Autodesk Inventor part; units mm, degrees
ref_plane "YZ Plane" through (0, 0, 0) normal (1, 0, 0) x (0, 1, 0)
ref_plane "XZ Plane" through (0, 0, 0) normal (0, 1, 0) x (-1, 0, 0)
ref_plane "XY Plane" through (0, 0, 0) normal (0, 0, 1) x (1, 0, 0)
sketch "Sketch1" plane through (0, 0, 0) normal (1, 0, 0) x (0, 1, 0)
  line L0 (55.2257, 58.6909) -> (-32.0868, 58.6909)
  line L1 (-32.0868, 58.6909) -> (-32.0868, -73.0716)
  line L2 (-32.0868, -73.0716) -> (55.2257, -73.0716)
  line L3 (55.2257, -73.0716) -> (55.2257, 58.6909)
  point P0 (0, 0)
  dimension "d0" = 131.7625
  dimension "d1" = 87.3125
extrude "Extrusion1" add sketch "Sketch1" along normal blind 31.75
sketch "Sketch2" plane through (0, -32.0868, -73.0716) normal (0, -1, 0) x (1, 0, 0)
  line L0 (31.75, 131.7625) -> (31.75, 0)
  line L1 (0, 131.7625) -> (0, 0)
  line L2 (28.575, 28.575) -> (3.175, 28.575)
  line L3 (3.175, 28.575) -> (3.175, 0)
  line L4 (3.175, 0) -> (28.575, 0)
  line L5 (28.575, 0) -> (28.575, 28.575)
  point P0 (0, 73.0716)
  point P1 (31.75, 28.575)
  dimension "d7" = 3.175
  dimension "d8" = 3.175
  dimension "d9" = 28.575
extrude "Extrusion2" cut sketch "Sketch2" against normal blind 87.3125
sketch "Sketch3" plane through (28.575, -32.0868, -44.4966) normal (0, 0, -1) x (-1, 0, 0)
  line L0 (0, 0) -> (0, 87.3125)
  line L1 (25.4, 0) -> (25.4, 87.3125)
  line L2 (0, 3.175) -> (25.4, 3.175)
  line L3 (25.4, 3.175) -> (25.4, 84.1375)
  line L4 (25.4, 84.1375) -> (0, 84.1375)
  line L5 (0, 84.1375) -> (0, 3.175)
  line L6 (0, 87.3125) -> (25.4, 87.3125)
  line L7 (25.4, 0) -> (0, 0)
  point P0 (28.575, 32.0868)
  point P1 (12.7, 84.1375)
  point P2 (12.7, 3.175)
  point P3 (0, 84.1375)
  point P4 (25.4, 3.175)
  dimension "d10" = 3.175
  dimension "d11" = 3.175
extrude "Extrusion3" cut sketch "Sketch3" against normal blind 47.625 contours L0 L4 L1 L2
sketch "Sketch4" plane through (0, -32.0868, -73.0716) normal (0, -1, 0) x (1, 0, 0)
  line L0 (3.175, 28.575) -> (28.575, 28.575)
  line L1 (25.4, 28.575) -> (6.35, 28.575)
  line L2 (6.35, 28.575) -> (6.35, 50.8)
  line L3 (6.35, 50.8) -> (25.4, 50.8)
  line L4 (25.4, 50.8) -> (25.4, 28.575)
  line L5 (31.75, 131.7625) -> (31.75, 0)
  circle A0 centre (16.7802, 41.275) radius 3.302
  point P0 (0, 73.0716)
  point P1 (15.875, 50.8)
  point P2 (15.875, 28.575)
  point P3 (25.4, 39.6875)
  point P4 (6.35, 28.575)
  dimension "d14" = 22.225
  dimension "d15" = 19.05
  dimension "d16" = 6.35
  dimension "d17" = 6.604
  dimension "d18" = 12.7
extrude "Extrusion4" cut sketch "Sketch4" against normal blind 1.5875
sketch "Sketch6" plane through (0, -30.4993, -73.0716) normal (0, -1, 0) x (1, 0, 0)
  circle A0 centre (16.7802, 41.275) radius 3.302
  circle A1 centre (16.7802, 41.275) radius 3.302
  point P0 (0, 73.0716)
extrude "Extrusion5" cut sketch "Sketch6" along normal mid plane 3.175
ref_plane "Work Plane2" through (0, 11.5695, -73.0716) normal (0, -1, 0) x (1, 0, 0)
mirror "Mirror1" about plane through (0, 11.5695, -73.0716) normal (0, -1, 0) of "Extrusion4"
mirror "Mirror2" about plane through (0, 11.5695, -73.0716) normal (0, -1, 0) of "Extrusion5"
fillet "Fillet1" radius 3.175 4 edges at (30.1625, -32.0868, -73.0716) (1.5875, -32.0868, -73.0716) (30.1625, 55.2257, -73.0716) (1.5875, 55.2257, -73.0716)
fillet "Fillet2" radius 3.175 2 edges at (15.875, -32.0868, 58.6909) (15.875, 55.2257, 58.6909)
fillet "Fillet3" radius 3.175 4 edges at (6.35, -31.293, -22.2716) (25.4, -31.293, -22.2716) (25.4, 54.432, -22.2716) (6.35, 54.432, -22.2716)
sketch "Sketch8" plane through (0, 0, 0) normal (-1, 0, 0) x (0, 0, 1)
  line L0 (-69.8966, 55.2257) -> (55.5159, 55.2257)
  line L1 (-73.0716, -28.9118) -> (-73.0716, 52.0507)
  arc A0 (31.0026, -12.8486) -> (30.8894, -18.4035) centre (28.5284, -15.5768) ccw
  arc A1 (36.1718, -17.4816) -> (36.1484, -13.6718) centre (36.1484, -15.5768) ccw
  line L2 (36.1484, -13.6718) -> (33.1356, -13.6718)
  line L3 (36.1718, -17.4816) -> (32.75, -17.6702)
  arc A2 (31.0026, -12.8486) -> (33.1356, -13.6718) centre (33.1356, -10.4968) ccw
  arc A3 (32.75, -17.6702) -> (30.8894, -18.4035) centre (32.9247, -20.8403) ccw
  line L4 (55.5159, -32.0868) -> (-69.8966, -32.0868)
  arc A4 (31.0026, 37.9514) -> (31.0026, 32.4951) centre (28.5284, 35.2232) ccw
  arc A5 (36.1484, 33.3182) -> (36.1484, 37.1282) centre (36.1484, 35.2232) ccw
  line L5 (36.1484, 37.1282) -> (33.1356, 37.1282)
  line L6 (36.1484, 33.3182) -> (33.1356, 33.3182)
  arc A6 (31.0026, 37.9514) -> (33.1356, 37.1282) centre (33.1356, 40.3032) ccw
  arc A7 (33.1356, 33.3182) -> (31.0026, 32.4951) centre (33.1356, 30.1432) ccw
  point P0 (0, 0)
  point P1 (31.6805, -13.6718)
  point P2 (31.5103, -17.7385)
  point P3 (31.8314, 36.8525)
  point P4 (31.2779, 32.7727)
  point P5 (31.6805, 37.1282)
  point P6 (31.6805, 33.3182)
  dimension "d57" = 3.81
  dimension "d58" = 7.366
  dimension "d59" = 3.175
  dimension "d60" = 101.6
  dimension "d61" = 109.22
  dimension "d63" = 0
  dimension "d77" = 101.6
  dimension "d78" = 109.22
  dimension "d79" = 50.8
  dimension "d80" = 20.0025
  dimension "d81" = 3.81
  dimension "d82" = 7.366
  dimension "d83" = 3.175
extrude "Extrusion7" cut sketch "Sketch8" against normal blind 6.4008
properties part number "cDAQ_Chassis_LowPolyPlaceholder"
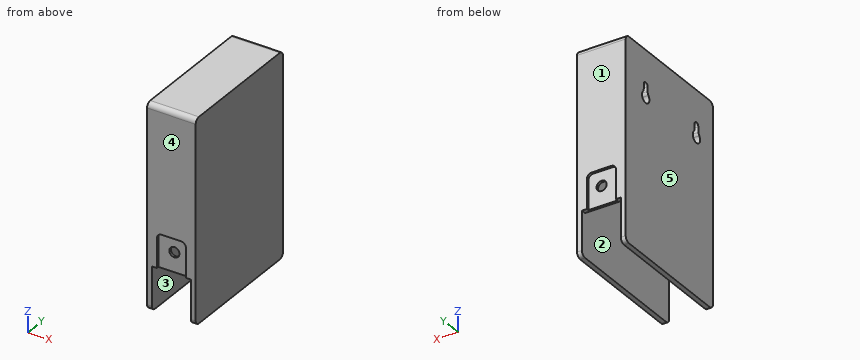
Read the model definition and answer for the solid it produces. Units are mm, in the model's axes. Face numbers are marked on the shaded views. A direction names the side the tool comes from. Round coordinates to 2 decimals unless told otherwise and drop trailing zeros. Write each loop counter-clockwise with the first axis right and the second up, starting at its lowest first coordinate (ties: lowest second). Pieces come first, ordered by that corner, then holes. Notation, with made-up numbers: M 7,69.25 L 38,69.25 A20 cw 38,96.25 Z; hole C 74,71 d6. An arc over 180 degrees is marked long. One line per item, written item: value.
Q1. Which of the six approach directions +Z, -Z, +X, -X, +Y, -Y give full straight-line access (tool end or side, diameter ignored) to the marked faces 1 and 2?
Data:
face 1: +Z, -Z, +X, -X, +Y
face 2: -Z
Q2. Flat-ended cylindrical pins translate along their axes: pin 1 Ø6 at (x, y) = (8.5, 10.5) entering from -Z; pin 2 Ø0.5 at (y, z) = (-31.5, -31) entering from -X; pin 3 Ø5.5 at (x, z) = (12.5, -36.5) entering from +Y; pin 4 Ø5.5 at (x, z) = (15, -35.5) entering from -Y. Find the tip coordinate at first contact, or state that the pin passes through.
Data:
pin 1: z = 3.13
pin 2: x = 0
pin 3: y = 53.64
pin 4: y = -30.5
Q3. Find section B-B on x = 16.5. Write down the section's boundary in (y, z) (3 decimals), plus the area to 3 significant figures.
Data:
outline: M -32.087,-22.272 L -30.499,-22.272 L -30.499,-28.507 L -28.912,-28.507 L -28.912,3.128 L 52.051,3.128 L 52.051,-28.507 L 53.638,-28.507 L 53.638,-22.272 L 55.226,-22.272 L 55.226,55.516 A3.175 ccw 52.051,58.691 L -28.912,58.691 A3.175 ccw -32.087,55.516 Z; M -30.499,-44.497 L -28.912,-44.497 L -28.912,-35.087 L -30.499,-35.087 Z; M 52.051,-44.497 L 53.638,-44.497 L 53.638,-35.087 L 52.051,-35.087 Z
area: 5,060 mm2
Q4. Find section C-C on z = -56.5. Write down the section's boundary in (x, y) (3 decimals), plus the area to 3 significant figures.
Data:
outline: M 0,-32.087 L 3.175,-32.087 L 3.175,55.226 L 0,55.226 Z; M 28.575,-32.087 L 31.75,-32.087 L 31.75,55.226 L 28.575,55.226 Z
area: 554 mm2
Q5. Find section A-A on z = -5.5. Write down the section's boundary in (x, y) (3 decimals).
Data:
outline: M 0,-32.087 L 31.75,-32.087 L 31.75,55.226 L 0,55.226 Z; hole M 3.175,-28.912 L 28.575,-28.912 L 28.575,52.051 L 3.175,52.051 Z
Q6. Find section D-D on y = 49.5. Write down the section's boundary in (x, z) (3 decimals).
Data:
outline: M 0,-73.072 L 3.175,-73.072 L 3.175,3.128 L 28.575,3.128 L 28.575,-73.072 L 31.75,-73.072 L 31.75,58.691 L 0,58.691 Z
Q7. For a pull along Y with two mould halves and no side action, classify the marked faces 3, 4 and 5 as +Y half, -Y half, draft (parallel to the pull), parting line (faces both ways), or undercut.
Data:
face 3: undercut
face 4: -Y half
face 5: draft
Q8. Straight lines are drawn through the part: line 1 (Y direction, x = 3, z = 28.5); line 2 (X direction, y = 0, z = -40.5) (3 decimals); line 3 (Y direction, x = 13, z = -41.5). For each, find the intervals that lie inside material, in ascending order. Write a range as [from, to].
Data:
line 1: [-32.09, -19.26], [-11.89, 31.54], [38.91, 55.23]
line 2: [0, 3.175], [28.575, 31.75]
line 3: [-30.5, -28.91], [52.05, 53.64]
